Could you check a few things on this model? Use its own coordinates, in mm. A direction names the side the tool comes from. Give positions to 0.01 mm unless a question says otherwise; leave off trailing zeros. Loops run counter-clockwise (first coordinate to the right, second up) from the corner with the lowest first, then second, coordinate; pieces in that order, holes last. Notation, with made-up numbers: M 8,32 L 32,32 A17 cw 32,38 Z; hole C 75,55 d1. An arc over 180 degrees is marked long. Return JSON: item names as keys, results as strings. Group by question number.
1. If we section it at B-B (z = 29): Write out the boundary of the cut face in (x, y), plus the area to 3 significant figures.
2. For faces 5 (the flat face through (-3, 2, -13)), 6 (the flat face through (-12, 0, -1)), which set-ups out of +Z, -Z, +X, -X, +Y, -Y let a thin tool reach every point of the face, with its end or its side?
3. If we mould it in two halves opening along X, with no side actions, what happens to faces 1 (the cylindrical face through (1.86, 1.97, 51.5)), 2 (the cylindrical face through (-35.17, 1.97, 0.33)), 3 (the cylindrical face through (-22.21, 1.97, 53.58)), 4 (the flat face through (-12, 4, -1))? For each: +X half, -X half, draft (parallel to the pull), parting line (faces both ways), or undercut.
4. Please list where these lines run through material, in increasing order: line 1 (X direction, y = 1.55, z = 0); line 2 (Z direction, x = 9, y = 2.15); line 3 (Z direction, x = 1, y = 1.6).
5. If we section it at C-C (y = 3.3): Write out the boundary of the cut face in (x, z).
6. If we section it at D-D (x = 17): Write out the boundary of the cut face in (y, z), plus the area to 3 significant figures.
7. For pin 1 (1.5 mm diameter, centred on x = -34, y = 3, fed in from -Z); pin 2 (1.2 mm diameter, centred on y = 1.5, z = -11.5, fed in from -X); pin 3 (1.2 mm diameter, centred on y = 1.5, z = -12.5, fed in from +X), each with a flat end and sliding along its axis, tell me the tip position at first contact or that it passes through.
8. If we section it at A-A (z = 0): Write out the boundary of the cut face in (x, y).
```python
from build123d import *

# Parameters (mm, degrees)
SKETCH_1_R          = 58
EXTRUDE_1_DEPTH     = 4
SKETCH_3_R          = 1.5
CUT_EXTRUDE_1_DEPTH = 50
CUT_EXTRUDE_2_DEPTH = 500


with BuildPart() as part:
    # 草图1 → 凸台-拉伸1 (new body)
    with BuildSketch(Plane(origin=(0, 0, 0), x_dir=(1, 0, 0), z_dir=(0, 1, 0))):
        with Locations(Location((0, 0, 0), (0, 0, 270))):
            Circle(SKETCH_1_R)
    extrude(amount=EXTRUDE_1_DEPTH)

    # 草图3 → 切除-拉伸1 (cut)
    with BuildSketch(Plane.XZ):
        with Locations(Location((1.793366497, -50, 0), (0, 0, 270))):
            Circle(SKETCH_3_R)
        with Locations(Location((-33.706633503, 0, 0), (0, 0, 270))):
            Circle(SKETCH_3_R)
        with Locations(Location((1.793366497, 50, 0), (0, 0, 270))):
            Circle(SKETCH_3_R)
        with Locations(Location((51.793366497, 0, 0), (0, 0, 270))):
            Circle(SKETCH_3_R)
    extrude(amount=-CUT_EXTRUDE_1_DEPTH, mode=Mode.SUBTRACT)

    # 草图4 → 切除-拉伸2 (cut)
    with BuildSketch(Plane(origin=(0, 4, 0), x_dir=(1, 0, 0), z_dir=(0, 1, 0))):
        Polygon((3, 9), (10, 9), (10, -31), (-10, -31), (-10, 9), (-3, 9), (-3, 17), (3, 17), align=None)
    extrude(amount=-CUT_EXTRUDE_2_DEPTH, mode=Mode.SUBTRACT)


solid = part.part
```
Answer:
{
 "1": {"outline": "M -50.23,0 L -10,0 L -10,4 L -50.23,4 Z; M 10,0 L 50.23,0 L 50.23,4 L 10,4 Z", "area": "322 mm²"},
 "2": {"face 5": "+Y, -Y", "face 6": "+Z, -Z, +X, -X, -Y"},
 "3": {"face 1": "undercut", "face 2": "undercut", "face 3": "parting line", "face 4": "draft"},
 "4": {"line 1": "x = -58 to -35.21, -32.21 to -10, 10 to 50.29, 53.29 to 58", "line 2": "z = -57.3 to -9, 31 to 57.3", "line 3": "z = -57.99 to -51.27, -48.73 to -17, 31 to 48.73, 51.27 to 57.99"},
 "5": {"outline": "C 0,0 d116; hole C -33.71,0 d3; hole M -10,-9 L -3,-9 L -3,-17 L 3,-17 L 3,-9 L 10,-9 L 10,31 L -10,31 Z; hole C 1.79,-50 d3; hole C 1.79,50 d3; hole C 51.79,0 d3"},
 "6": {"outline": "M 0,-55.45 L 4,-55.45 L 4,55.45 L 0,55.45 Z", "area": "444 mm²"},
 "7": {"pin 1": "stops at z = -47.52", "pin 2": "stops at x = -56.97", "pin 3": "stops at x = 56.77"},
 "8": {"outline": "M -58,0 L -35.21,0 L -35.21,4 L -58,4 Z; M -32.21,0 L -10,0 L -10,4 L -32.21,4 Z; M 10,0 L 50.29,0 L 50.29,4 L 10,4 Z; M 53.29,0 L 58,0 L 58,4 L 53.29,4 Z"}
}
